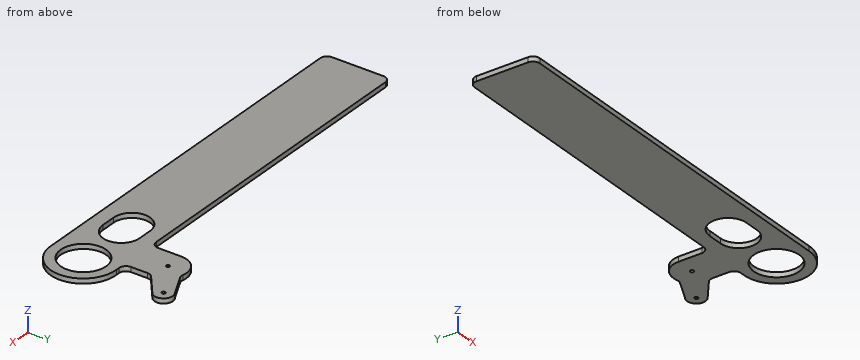
```python
from build123d import *

# Parameters (mm, degrees)
F0_R     = 16.35
F0_R_2   = 1.25
F1_DEPTH = 3.5


with BuildPart() as f1:
    # F0 (on Top) → F1 (new body)
    with BuildSketch(Plane.XY):
        with BuildLine():
            ThreePointArc((-118.087944, -18.483081), (-116.623477, -22.018615), (-113.087944, -23.483081))
            Line((-113.087944, -23.483081), (154.055671, -23.483081))
            ThreePointArc((154.055671, -23.483081), (177.739071, 0.200008), (153.688095, 23.509721))
            ThreePointArc((153.688095, 23.509721), (153.629408, 23.508687), (153.570713, 23.508343))
            Line((153.570713, 23.508343), (151.117662, 23.508343))
            ThreePointArc((151.117662, 23.508343), (147.582128, 24.972809), (146.117662, 28.508343))
            Line((146.117662, 28.508343), (146.117662, 40.43658))
            ThreePointArc((146.117662, 40.43658), (146.619244, 42.619292), (148.023355, 44.364081))
            Line((148.023355, 44.364081), (162.493134, 55.764192))
            Line((162.493134, 55.764192), (163.489272, 56.549006))
            ThreePointArc((163.489272, 56.549006), (163.978244, 65.5632), (155.014432, 66.633185))
            Line((155.014432, 66.633185), (139.121962, 58.817696))
            ThreePointArc((139.121962, 58.817696), (137.471638, 58.335528), (135.755552, 58.440901))
            ThreePointArc((135.755552, 58.440901), (124.215423, 55.867), (119.134148, 45.190849))
            Line((119.134148, 45.190849), (119.134148, 28.508343))
            ThreePointArc((119.134148, 28.508343), (117.669682, 24.972809), (114.134148, 23.508343))
            Line((114.134148, 23.508343), (-113.087944, 23.508343))
            ThreePointArc((-113.087944, 23.508343), (-116.623477, 22.043877), (-118.087944, 18.508343))
            Line((-118.087944, 18.508343), (-118.087944, -18.483081))
        make_face()
        with BuildLine():
            ThreePointArc((105.981351, -13.13), (92.851351, 0), (105.981351, 13.13))
            Line((105.981351, 13.13), (116.481351, 13.13))
            ThreePointArc((116.481351, 13.13), (129.611351, 0), (116.481351, -13.13))
            Line((116.481351, -13.13), (105.981351, -13.13))
        make_face(mode=Mode.SUBTRACT)
        with Locations((154.055671, 0.016919)):
            Circle(F0_R, mode=Mode.SUBTRACT)
        with Locations((132.625611, 45.316919)):
            Circle(F0_R_2, mode=Mode.SUBTRACT)
        with Locations((158.925611, 61.316919)):
            Circle(F0_R_2, mode=Mode.SUBTRACT)
        with BuildLine():
            Line((163.489272, 56.549006), (162.493134, 55.764192))
            ThreePointArc((162.493134, 55.764192), (163.010096, 56.132618), (163.489272, 56.549006))
        make_face()
    extrude(amount=F1_DEPTH)


solid = f1.part
```
Source: CAD feature listing. Evaluate the final solid. Frame: model axes, mm. Round coordinates to 2 decimals unless told otherwise and drop trailing zeros. Order: outer loops, then holes, each group sorted by start corner. A loop starts at its lowest first (then second) coordinate and runs counter-clockwise, first axis right, second up. Notation, with made-up numbers: (-26, 12) -> (7, 12) arc R26 ccw to (7, 32) -> close; hole circle Ø10 at (8.5, 4.5). An arc over 180 degrees is marked (long way). Use CSV: the item, a comma, the result in double quotes.
(1) Section A-A on y = -6. Return the cut outline in (x, z).
Report:
outline,"(-118.09, 0) -> (94.3, 0) -> (94.3, 3.5) -> (-118.09, 3.5) -> close; (128.16, 0) -> (138.85, 0) -> (138.85, 3.5) -> (128.16, 3.5) -> close; (169.26, 0) -> (176.96, 0) -> (176.96, 3.5) -> (169.26, 3.5) -> close"
(2) Section B-B on z = 1. Return the cut outline in (x, y).
Report:
outline,"(-118.09, -18.48) arc R5 ccw to (-113.09, -23.48) -> (154.06, -23.48) arc R23.5 ccw (long way) to (153.69, 23.51) arc R4.99 cw to (153.57, 23.51) -> (151.12, 23.51) arc R5 cw to (146.12, 28.51) -> (146.12, 40.44) arc R5 cw to (148.02, 44.36) -> (162.49, 55.76) arc R6.6 ccw to (163.49, 56.55) arc R6.6 ccw to (155.01, 66.63) -> (139.12, 58.82) arc R5 cw to (135.76, 58.44) arc R13.49 ccw to (119.13, 45.19) -> (119.13, 28.51) arc R5 cw to (114.13, 23.51) -> (-113.09, 23.51) arc R5 ccw to (-118.09, 18.51) -> close; hole (105.98, -13.13) -> (116.48, -13.13) arc R13.13 ccw to (116.48, 13.13) -> (105.98, 13.13) arc R13.13 ccw to start; hole circle Ø2.5 at (132.63, 45.32); hole circle Ø32.7 at (154.06, 0.02); hole circle Ø2.5 at (158.93, 61.32)"
(3) First-contact query: pin 1 Ø1.8 at (x, z) = (110.5, 1) entering from +Y; pin 2 Ø1 at (y, z) = (37, 2.5) entering from +X. Flat tips, straight axial feed; report the tip coordinate or a pass-through.
Report:
pin 1,"y = 23.51"
pin 2,"x = 146.12"
(4) Section C-C on x = 73. Return the cut outline in (y, z), and give its area (3 significant figures).
Report:
outline,"(-23.48, 0) -> (23.51, 0) -> (23.51, 3.5) -> (-23.48, 3.5) -> close"
area,"164 mm^2"
(5) Ray query, L1, parallel to Y at x = 162.5, z = 2.7; L2, parallel to Y at x = 112, z = 3.2; L3, parallel to Y at x = 156, z = 1.9. Return the intervals inside material, ascending.
Report:
L1,"-21.98 to -13.98, 14.02 to 22.02, 55.77 to 66.87"
L2,"-23.48 to -13.13, 13.13 to 23.51"
L3,"-23.42 to -16.22, 16.25 to 23.45, 50.65 to 67.23"
